Verification items for the finished model (mm, model axes). A direction names the side the tool comes from. Round coordinates to 2 decimals unless told otherwise and drop trailing zeros. Order: outer loops, then holes, each group sorted by start corner. A loop starts at its lowest first (then second) coordinate and runs counter-clockwise, first axis right, second up. Notation, with made-up numbers: (61, 51) -> (114, 51) arc R24 cw to (114, 75) -> close; hole circle Ø10 at (57.25, -38). An arc over 180 degrees is marked (long way). Return JSON: item names as keys, results as strings. Group by question number.
1) Scan lines: L1, parallel to Z at x = 1.75, y = 28.5; L2, parallel to Z at x = 4, y = 33; L3, parallel to Y at x = 4.5, z = -85.5. Record each from-to range of solid material in increasing order.
2) Tool access check on faces 4 (the flat face through (6, 38, -43.18)), 5 (the flat face through (6, 24, 42.999)), 6 (the flat face through (6.8, 25, 77.6)). Record the directions out of +Z, -Z, +X, -X, +Y, -Y that give a thin tool (end or side, any length) a straight path to the whole face; none if there is none.
3) Section check C-C on y = 4.5. Enter the section's corners in (x, z), plus the area to 3 significant figures.
4) Draft check along Z on faces 1 (the flat face through (6, 38, 2.54)), 2 (the flat face through (0, 14, 1)), 3 (the flat face through (6.261, 24.083, -97.914)). Enter one of: pulls with the +Z half, pulls with the -Z half, needs draft (parallel to the pull), parting line crosses it, or undercut.
5) Section check A-A on x = 2. Enter the section's corners in (y, z) (1 decimal), plus the area to 3 significant figures.
6) Section check B-B on z = 25.5. Enter the section's corners in (x, y).
7) Depth check by flat-ended pin: pin 1 (4 mm diameter, centred on x = 8, y = 28.5, fed in from +Z); pin 2 (4 mm diameter, centred on x = 3.5, y = 24.5, fed in from +Z); pin 3 (1.5 mm diameter, centred on x = 11, y = 43, fed in from -Z); pin 4 (8 mm diameter, centred on y = 23, z = 33.5, fed in from -X). Enter the tip coordinate at first touch or a pass-through.
8) Section check D-D on y = 18.5. Enter the section's corners in (x, z), plus the area to 3 significant figures.
```python
from build123d import *

# Parameters (mm, degrees)
BOSS_EXTRUDE1_DEPTH = 12.7
CUT_EXTRUDE1_DEPTH  = 71.842048969
CUT_EXTRUDE2_REACH  = 120.838
FILLET1_R           = 1.5875


with BuildPart() as part:
    # Sketch1 → Boss-Extrude1 (new body)
    with BuildSketch(Plane(origin=(0, 0, 0), x_dir=(0, 0, -1), z_dir=(1, 0, 0))):
        with BuildLine():
            Line((-55.88, 50.8), (-106.68, 0))
            Line((-106.68, 0), (106.68, 0))
            Line((106.68, 0), (88.9, 48.850148518))
            Line((88.9, 48.850148518), (88.9, 12.7))
            Line((88.9, 12.7), (50.8, 12.7))
            Line((50.8, 12.7), (50.8, 50.8))
            Line((50.8, 50.8), (43.18, 50.8))
            Line((43.18, 50.8), (43.18, 25.4))
            ThreePointArc((43.18, 25.4), (20.32, 2.54), (-2.54, 25.4))
            Line((-2.54, 25.4), (-2.54, 50.8))
            Line((-2.54, 50.8), (-55.88, 50.8))
        make_face()
    extrude(amount=BOSS_EXTRUDE1_DEPTH)

    # Sketch2 → Cut-Extrude1 (cut, along a direction that is not the sketch's normal)
    with BuildSketch(Plane.XZ):
        Polygon((0, 106.68), (12.7, 106.68), (12.7, 99.06), align=None)
    extrude(amount=-CUT_EXTRUDE1_DEPTH, dir=(0, -0.7071067811865438, 0.7071067811865512), mode=Mode.SUBTRACT)

    # Sketch3 → Cut-Extrude2 (cut, up to next)
    with BuildSketch(Plane(origin=(12.7, 0, 0), x_dir=(0, 0, -1), z_dir=(1, 0, 0)), mode=Mode.PRIVATE) as cut_extrude2_sk1:
        Polygon((-42.999487758, 12.7), (-68.399487758, 12.7), (-42.999487758, 38.1), align=None)
    cut_extrude2_tool1 = extrude(cut_extrude2_sk1.sketch, amount=-CUT_EXTRUDE2_REACH, mode=Mode.PRIVATE) & part.part
    # Sketch3 → Cut-Extrude2 (cut, up to next)
    with BuildSketch(Plane(origin=(12.7, 0, 0), x_dir=(0, 0, -1), z_dir=(1, 0, 0)), mode=Mode.PRIVATE) as cut_extrude2_sk2:
        Polygon((-15.24, 23.040512242), (-30.299487758, 38.1), (-30.299487758, 12.7), (-15.24, 12.7), align=None)
    cut_extrude2_tool2 = extrude(cut_extrude2_sk2.sketch, amount=-CUT_EXTRUDE2_REACH, mode=Mode.PRIVATE) & part.part
    add(cut_extrude2_tool1.solids().sort_by_distance((12.7, 21.166667, 51.466154))[0], mode=Mode.SUBTRACT)
    add(cut_extrude2_tool2.solids().sort_by_distance((12.7, 22.163912, 23.827312))[0], mode=Mode.SUBTRACT)

    # Fillet1
    fillet1_edges = [part.edges().sort_by_distance(p)[0] for p in [
        (6.35, 12.7, 42.999487758),
        (6.35, 12.7, 68.399487758),
        (6.35, 38.1, 42.999487758),
        (6.35, 23.040512242, 15.24),
        (6.35, 12.7, 15.24),
        (6.35, 12.7, 30.299487758),
        (6.35, 38.1, 30.299487758),
    ]]
    fillet(fillet1_edges, radius=FILLET1_R)


solid = part.part
```
Check result:
{
 "1": {"L1": "-96.31 to -88.9, -50.8 to -43.18, 2.54 to 20.7, 30.3 to 43, 52.6 to 77.13", "L2": "-94.67 to -88.9, -50.8 to -43.18, 2.54 to 25.2, 30.3 to 43, 48.1 to 71.28", "L3": "0 to 12.7"},
 "2": {"face 4": "+X, -X, +Y", "face 5": "+X, -X", "face 6": "+Z, +X, +Y"},
 "3": {"outline": "(0, -105.04) -> (12.7, -105.04) -> (12.7, -29.58) -> (0, -29.58) -> close; (0, -11.06) -> (12.7, -11.06) -> (12.7, 94.56) -> (0, 102.18) -> close", "area": "2,350 mm^2"},
 "4": {"face 1": "undercut", "face 2": "needs draft", "face 3": "pulls with the -Z half"},
 "5": {"outline": "(0, -106.7) -> (48.9, -88.9) -> (12.7, -88.9) -> (12.7, -50.8) -> (50.8, -50.8) -> (50.8, -43.2) -> (25.4, -43.2) arc R22.9 cw to (25.4, 2.5) -> (50.8, 2.5) -> (50.8, 54.7) -> (0, 105.5) -> close; hole (12.7, 16.8) arc R1.6 ccw to (14.3, 15.2) -> (22.4, 15.2) arc R1.6 ccw to (23.5, 15.7) -> (35.4, 27.6) arc R1.6 ccw to (34.3, 30.3) -> (14.3, 30.3) arc R1.6 ccw to (12.7, 28.7) -> close; hole (12.7, 44.6) arc R1.6 ccw to (14.3, 43) -> (34.3, 43) arc R1.6 ccw to (35.4, 45.7) -> (15.4, 65.7) arc R1.6 ccw to (12.7, 64.6) -> close", "area": "5,000 mm^2"},
 "6": {"outline": "(0, 0) -> (12.7, 0) -> (12.7, 12.7) -> (0, 12.7) -> close; (0, 33.3) -> (12.7, 33.3) -> (12.7, 50.8) -> (0, 50.8) -> close"},
 "7": {"pin 1": "z = 75.71", "pin 2": "z = 82.41", "pin 3": "z = -91.3", "pin 4": "x = 0"},
 "8": {"outline": "(0, -99.95) -> (12.7, -99.95) -> (12.7, -88.9) -> (0, -88.9) -> close; (0, -50.8) -> (12.7, -50.8) -> (12.7, -42.11) -> (0, -42.11) -> close; (0, 1.47) -> (12.7, 1.47) -> (12.7, 15.24) -> (0, 15.24) -> close; (0, 30.3) -> (12.7, 30.3) -> (12.7, 43) -> (0, 43) -> close; (0, 62.6) -> (12.7, 62.6) -> (12.7, 80.56) -> (0, 88.18) -> close", "area": "863 mm^2"}
}
